Model file for the job. Use its own axes, mm. A direction names the side the tool comes from. Coordinates: 2 decimals unless noted, no trailing zeros. Order: outer loops, then holes, each group sorted by start corner. A loop starts at its lowest first (then second) coordinate and runs counter-clockwise, first axis right, second up. Notation, with made-up numbers: M 38,68 L 58,68 A24 cw 58,101 Z; hole C 30,5 d7. An arc over 180 degrees is marked long. Return JSON: item names as keys, results as strings.
```python
from build123d import *

# Parameters (mm, degrees)
F0_R     = 4.4
F1_DEPTH = 12
F2_R     = 7.5
F2_R_2   = 4.4
F3_DEPTH = 3
F5_SIZE  = 1


# Not quite as in the source:
# - a fillet or chamfer that OpenCascade refuses, or shapes differently, is made with other operations: its cross-section is extruded or revolved along the edge and cut away or added


with BuildPart() as f1:
    # F0 (on Front) → F1 (new body)
    with BuildSketch(Plane.XZ):
        Circle(F0_R)
    extrude(amount=F1_DEPTH)

    # F2 (on face) → F3 (join)
    with BuildSketch(Plane.XZ.offset(12)):
        Circle(F2_R)
        Circle(F2_R_2, mode=Mode.SUBTRACT)
        Circle(F2_R)
    extrude(amount=F3_DEPTH)

    # F4: fillet of radius 5 on 1 edges, made by hand

    # F4_s1 → F4_t2 (revolve, cut)
    with BuildSketch(Plane.XY):
        with BuildLine():
            ThreePointArc((7.5, -12), (5.6560370926, -14.1833001327), (2.917424305, -15))
            Line((2.917424305, -15), (7.5, -15))
            Line((7.5, -15), (7.5, -12))
        make_face()
    revolve(axis=Axis((0, -15, 0), (0, -1, 0)), mode=Mode.SUBTRACT)

    # F5
    f5_edges = [f1.edges().sort_by_distance(p)[0] for p in [
        (-4.4, 0, 0),
    ]]
    chamfer(f5_edges, length=F5_SIZE)


solid = f1.part
```
Item 1: Drop flat-ended pins along their axis: pin 1 Ø4 at (x, y) = (-3.5, -5.5) entering from -Z; pin 2 Ø1 at (y, z) = (-6.5, 2) entering from -X. Give the stop position or say it passes through.
Check result:
{"pin 1": "stops at z = -4.14", "pin 2": "stops at x = -4.14"}
Item 2: Wall check: line 1 (Y direction, x = -4.75, z = 1.5); line 2 (Z direction, x = 3, y = -3.75); line 3 (X direction, y = -10, z = -2). Give the ranges that are in metal, low to high.
Check result:
{"line 1": "y = -14.55 to -12", "line 2": "z = -3.22 to 3.22", "line 3": "x = -3.92 to 3.92"}
Item 3: Saw through at A-A (y = -7.25). Write the cut outline in (x, z).
Check result:
{"outline": "C 0,0 d8.8"}
Item 4: 3-axis set-ups, long thin cutter, end or side, ignore diameter. For faces 1 (the cylindrical face through (4.197, -6.423, 1.322)), 2 (the flat face through (0, 0, 0)): which of +Z, -Z, +X, -X, +Y, -Y reach the whole face in a straight line?
Check result:
{"face 1": "+Y", "face 2": "+Z, -Z, +X, -X, +Y"}
